Read the model definition and answer for the solid it produces. Units are mm, in the model's axes. Face numbers are marked on the shaded views. Give positions to 0.01 mm unless a question says otherwise; leave off trailing zeros. Loops run counter-clockwise (first coordinate to the right, second up) from the corner with the lowest first, then second, coordinate; pieces in that order, holes last. Notation, with made-up numbers: (37, -28.75) - (77, -28.75) arc R20 cw to (77, -14.75) - close; hole circle Ø9 at (0, 87.5). An arc over 180 degrees is marked (long way). Write item = value, one per line.
```python
from build123d import *

# Parameters (mm, degrees)
SKETCH_3_R               = 5
CUT_EXTRUDE_1_DEPTH      = 164.859696082
SKETCH_4_R               = 10
CUT_EXTRUDE_2_DEPTH      = 10
CUT_EXTRUDE_START        = -5
CUT_EXTRUDE_3_DEPTH      = 5
CHAMFER_2_SIZE           = 2
SKETCH_7_W               = 8
SKETCH_7_H               = 20
CUT_EXTRUDE_7_DEPTH      = 7.5
PATTERN_CIRCULAR_1_COUNT = 6


with BuildPart() as part:
    # Эскиз1 → Повернуть1 (revolve)
    with BuildSketch(Plane.XY, mode=Mode.PRIVATE) as revolve_1_sk:
        Polygon((115, 23.777702661), (77.5, 23.777702661), (77.5, 43.777702661), (110, 43.777702661), (115, 40.890951315), align=None)
    revolve(revolve_1_sk.sketch.rotate(Axis((0, 147.550331696, 0), (0, -1, 0)), 90), axis=Axis((0, 147.550331696, 0), (0, -1, 0)))

    # Эскиз3 → Вырез-Вытянуть1 (cut, through all)
    with BuildSketch(Plane(origin=(0, 43.777702661, 0), x_dir=(1, 0, 0), z_dir=(0, 1, 0))):
        with Locations(Location((86.602540378, -50, 0), (0, 0, 270))):
            Circle(SKETCH_3_R)
    extrude(amount=-CUT_EXTRUDE_1_DEPTH, mode=Mode.SUBTRACT)

    # Эскиз4 → Вырез-Вытянуть2 (cut)
    with BuildSketch(Plane.XZ.offset(-23.777702661)):
        with Locations(Location((86.602540378, 50, 0), (0, 0, 270))):
            Circle(SKETCH_4_R)
    extrude(amount=-CUT_EXTRUDE_2_DEPTH, mode=Mode.SUBTRACT)

    # Эскиз5 → Вырез-Вытянуть3 (cut)
    with BuildSketch(Plane(origin=(0, 43.777702661, 0), x_dir=(1, 0, 0), z_dir=(0, 1, 0)).offset(CUT_EXTRUDE_START)):
        with BuildLine():
            Line((91.602540378, -41.339745962), (136.199116664, -67.087591285))
            Line((136.199116664, -67.087591285), (126.755895542, -84.729555796))
            Line((126.755895542, -84.729555796), (81.602540378, -58.660254038))
            ThreePointArc((81.602540378, -58.660254038), (77.942286341, -45), (91.602540378, -41.339745962))
        make_face()
    extrude(amount=CUT_EXTRUDE_3_DEPTH, mode=Mode.SUBTRACT)

    # Фаска2
    chamfer_2_edges = [part.edges().sort_by_distance(p)[0] for p in [
        (0, 23.777702661, -115),
    ]]
    chamfer(chamfer_2_edges, length=CHAMFER_2_SIZE)

    # Эскиз7 → Вырез-Вытянуть7 (cut, symmetric)
    with BuildSketch(Plane.XY):
        with Locations((-111, 33.777702661)):
            Rectangle(SKETCH_7_W, SKETCH_7_H)
    cut_extrude_7 = extrude(amount=CUT_EXTRUDE_7_DEPTH, both=True, mode=Mode.SUBTRACT)

    # Круговой массив1: Вырез-Вытянуть7 ×6 about axis
    pattern_circular_1_axis = Axis((0, 0, 0), (0, 1, 0))
    for i in range(1, PATTERN_CIRCULAR_1_COUNT):
        add(cut_extrude_7.rotate(pattern_circular_1_axis, i * 360 / PATTERN_CIRCULAR_1_COUNT), mode=Mode.SUBTRACT)


solid = part.part
```
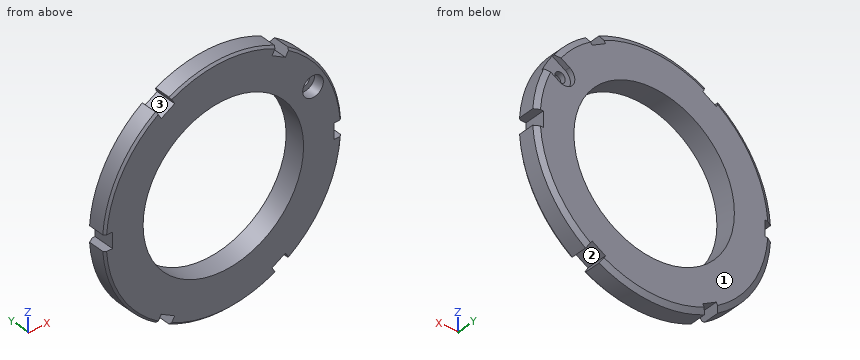
1) A cutting plane is placed at C-C on y = 30.5. Determine the outline of the cut face in (x, z), then the cut area to 3 significant figures.
Output:
outline = (-114.76, -7.5) arc R115 ccw to (-63.87, -95.63) - (-60, -88.91) - (-47, -96.41) - (-50.88, -103.13) arc R115 ccw to (50.88, -103.13) - (47, -96.41) - (60, -88.91) - (63.87, -95.63) arc R115 ccw to (114.76, -7.5) - (107, -7.5) - (107, 7.5) - (114.76, 7.5) arc R115 ccw to (63.87, 95.63) - (60, 88.91) - (47, 96.41) - (50.88, 103.13) arc R115 ccw to (-50.88, 103.13) - (-47, 96.41) - (-60, 88.91) - (-63.87, 95.63) arc R115 ccw to (-114.76, 7.5) - (-107, 7.5) - (-107, -7.5) - close; hole circle Ø155 at (0, 0); hole circle Ø20 at (86.6, 50)
area = 21,700 mm²
2) Find the intervals of material crossed by probe 1 along X at (y, z) = (38, 0); probe 2 along X at (y, z) = (31.25, 50); probe 3 along Z at (x, y) = (50.5, 35.75), in increasing order.
Output:
probe_1 = -107 to -77.5, 77.5 to 107
probe_2 = -103.56 to -59.21, 59.21 to 76.6, 96.6 to 103.56
probe_3 = -103.32 to -102.47, -94.4 to -58.79, 58.79 to 94.4, 102.47 to 103.32
3) Each of these flat-tipped pins is pushed along its axis until it touches: P1, Ø18, axis at x = 86.6, z = 50, coming from the +Y side; P2, Ø11.5, axis at x = 86.6, z = 50, coming from the -Y side; P3, Ø6, axis at y = 39, z = 16.5, coming from the +X side. Where does it stop, or does it pass through?
Output:
P1 = 38.78
P2 = 33.78
P3 = 114.2
4) A cutting plane is placed at B-B on x = 0. Determine the outline of the cut face in (y, z).
Output:
outline = (23.78, -113) - (25.78, -115) - (40.89, -115) - (43.78, -110) - (43.78, -77.5) - (23.78, -77.5) - close; (23.78, 77.5) - (43.78, 77.5) - (43.78, 110) - (40.89, 115) - (25.78, 115) - (23.78, 113) - close
5) A cutting plane is placed at A-A on z = 0. Determine the outline of the cut face in (x, y).
Output:
outline = (-107, 23.78) - (-77.5, 23.78) - (-77.5, 43.78) - (-107, 43.78) - close; (77.5, 23.78) - (107, 23.78) - (107, 43.78) - (77.5, 43.78) - close
6) The mould has two halves that part along Z. Classify the marked faces 1, 2 and 3: pulls with the +Z half, pulls with the -Z half, needs draft (parallel to the pull), parting line crosses it, or undercut.
Output:
face_1 = needs draft
face_2 = undercut
face_3 = undercut
